```python
from build123d import *

# Parameters (mm, degrees)
SKETCH1_W           = 50
SKETCH1_H           = 40
BOSS_EXTRUDE1_DEPTH = 10
SKETCH2_W           = 10
SKETCH2_H           = 40
BOSS_EXTRUDE2_DEPTH = 21
SKETCH4_W           = 10
SKETCH4_H           = 40
BOSS_EXTRUDE3_DEPTH = 10
SKETCH5_W           = 40
SKETCH5_H           = 10
BOSS_EXTRUDE4_DEPTH = 40
SKETCH6_R           = 7.5
SKETCH6_R_2         = 2.5
CUT_EXTRUDE1_DEPTH  = 40
SKETCH7_R           = 2.5
CUT_EXTRUDE2_DEPTH  = 77.032887621
SKETCH8_R           = 2.5
SKETCH8_R_2         = 2.34
BOSS_EXTRUDE5_DEPTH = 10


with BuildPart() as part:
    # Sketch1 → Boss-Extrude1 (new body)
    with BuildSketch(Plane(origin=(0, 0, 0), x_dir=(1, 0, 0), z_dir=(0, 1, 0))):
        with Locations((25, 20)):
            Rectangle(SKETCH1_W, SKETCH1_H)
    extrude(amount=BOSS_EXTRUDE1_DEPTH)

    # Sketch2 → Boss-Extrude2 (add)
    with BuildSketch(Plane.XZ):
        with Locations((5, -20)):
            Rectangle(SKETCH2_W, SKETCH2_H)
    extrude(amount=BOSS_EXTRUDE2_DEPTH)

    # Sketch4 → Boss-Extrude3 (add)
    with BuildSketch(Plane.XZ.offset(21)):
        with Locations((5, -20)):
            Rectangle(SKETCH4_W, SKETCH4_H)
    extrude(amount=BOSS_EXTRUDE3_DEPTH)

    # Sketch5 → Boss-Extrude4 (add)
    with BuildSketch(Plane(origin=(10, 0, 0), x_dir=(0, 0, -1), z_dir=(1, 0, 0))):
        with Locations((20, -26)):
            Rectangle(SKETCH5_W, SKETCH5_H)
    extrude(amount=BOSS_EXTRUDE4_DEPTH)

    # Sketch6 → Cut-Extrude1 (cut)
    with BuildSketch(Plane.ZY):
        with Locations((-20, -10.5)):
            Circle(SKETCH6_R)
        with Locations((-34.28, -10.5)):
            Circle(SKETCH6_R_2)
        with Locations((-5.72, -10.5)):
            Circle(SKETCH6_R_2)
    extrude(amount=-CUT_EXTRUDE1_DEPTH, mode=Mode.SUBTRACT)

    # Sketch7 → Cut-Extrude2 (cut, through all)
    with BuildSketch(Plane.XZ.offset(31)):
        with Locations(Location((18, -8, 0), (0, 0, 270))):
            Circle(SKETCH7_R)
        with Locations(Location((42, -8, 0), (0, 0, 270))):
            Circle(SKETCH7_R)
        with Locations(Location((18, -32, 0), (0, 0, 270))):
            Circle(SKETCH7_R)
        with Locations(Location((42, -32, 0), (0, 0, 270))):
            Circle(SKETCH7_R)
    extrude(amount=-CUT_EXTRUDE2_DEPTH, mode=Mode.SUBTRACT)

    # Sketch8 → Boss-Extrude5 (add)
    # profile 1 of 2: a face of its own
    with BuildSketch(Plane.ZY):
        with Locations((-34.28, -10.5)):
            Circle(SKETCH8_R)
        with Locations((-34.28, -10.5)):
            Circle(SKETCH8_R_2, mode=Mode.SUBTRACT)
    # profile 2 of 2: a face of its own
    with BuildSketch(Plane.ZY):
        with Locations((-5.72, -10.5)):
            Circle(SKETCH8_R)
        with Locations((-5.72, -10.5)):
            Circle(SKETCH8_R_2, mode=Mode.SUBTRACT)
    extrude(amount=-BOSS_EXTRUDE5_DEPTH)


solid = part.part
```
Part model, mm, in its own coordinate system. A direction names the side the tool comes from. Round coordinates to 2 decimals unless told otherwise and drop trailing zeros. Order: outer loops, then holes, each group sorted by start corner. A loop starts at its lowest first (then second) coordinate and runs counter-clockwise, first axis right, second up. Notation, with made-up numbers: M 26.5,-12.75 L 38.5,-12.75 A14 cw 38.5,7.25 Z; hole C 81,-31 d9. An arc over 180 degrees is marked long. Put each result on its own line as item: value. Start each with the question number.
1. Slice it at B-B on x = 18. List the corners of the cut face in (y, z).
2. Slice it at D-D on y = -10.5. List the corners of the cut face in (x, z).
3. Drop flat-ended pins along their axis: pin 1 (4 mm diameter, centred on x = 7.5, y = 2, fed in from +Z); pin 2 (19.5 mm diameter, centred on y = -10.5, z = -20, fed in from +X). Give the stop position or say it passes through.
4. Slice it at C-C on z = -20. List the corners of the cut face in (x, y), then the cut area to 3 significant figures.
5. Slice it at A-A on y = -27.5. List the corners of the cut face in (x, z), then the cut area to 3 significant figures.
6. Two-plate mould, pull along X, no slides. Class faces 3 (the face through (0, -10, -11)), 4 (the face through (25, 10, -20)), 5 (the face through (39.56, -26.07, -7.46)): +X half, -X half, draft (parallel to the pull), parting line (faces both ways), or undercut.
7. Drill centre lines: probe 1 along X at (y, z) = (-26, -8); probe 2 along Y at (x, z) = (22, -29.5); probe 3 along Z at (x, y) = (4, -10). Where is each one in solid material? Low to high. Write a range as [from, to].
8. Tool access for faces 1 (the face through (50, -26, -20)), 2 (the face through (10, -3, -16)): list every direction of +Z, -Z, +X, -X, +Y, -Y with a clear straight run to the whole face (end or side of a thin tool).
Findings:
1. outline: M -31,-40 L -21,-40 L -21,-34.5 L -31,-34.5 Z; M -31,-29.5 L -21,-29.5 L -21,-10.5 L -31,-10.5 Z; M -31,-5.5 L -21,-5.5 L -21,0 L -31,0 Z; M 0,-40 L 10,-40 L 10,-34.5 L 0,-34.5 Z; M 0,-29.5 L 10,-29.5 L 10,-10.5 L 0,-10.5 Z; M 0,-5.5 L 10,-5.5 L 10,0 L 0,0 Z
2. outline: M 0,-40 L 10,-40 L 10,-36.62 L 0,-36.62 Z; M 0,-31.94 L 10,-31.94 L 10,-27.5 L 0,-27.5 Z; M 0,-12.5 L 10,-12.5 L 10,-8.06 L 0,-8.06 Z; M 0,-3.38 L 10,-3.38 L 10,0 L 0,0 Z
3. pin 1: z = 0
3. pin 2: x = 10
4. outline: M 0,-31 L 50,-31 L 50,-21 L 10,-21 L 10,-18 L 0,-18 Z; M 0,-3 L 10,-3 L 10,0 L 50,0 L 50,10 L 0,10 Z
4. area: 1,060 mm2
5. outline: M 0,-40 L 50,-40 L 50,0 L 0,0 Z; hole C 18,-32 d5; hole C 18,-8 d5; hole C 42,-32 d5; hole C 42,-8 d5
5. area: 1,920 mm2
6. face 3: -X half
6. face 4: draft
6. face 5: undercut
7. probe 1: [0, 15.5], [20.5, 39.5], [44.5, 50]
7. probe 2: [-31, -21], [0, 10]
7. probe 3: [-40, -36.57], [-31.99, -27.48], [-12.52, -8.01], [-3.43, 0]
8. face 1: +Z, -Z, +X, +Y, -Y
8. face 2: +Z, -Z, +X
